from build123d import *

# Parameters (mm, degrees)
SKETCH_R     = 9
SKETCH_R_2   = 4
PAD_DEPTH    = 10
SKETCH001_R  = 2.5
POCKET_DEPTH = 10.001
CHAMFER_SIZE = 3


with BuildPart() as part:
    # Sketch → Pad (new body)
    with BuildSketch(Plane.XZ):
        with BuildLine():
            Line((0, 0), (0, 25))
            Line((0, 25), (-10, 25))
            Line((-10, 25), (-10, 55))
            Line((-10, 55), (0, 55))
            Line((0, 55), (0, 80))
            Line((0, 80), (-10, 80))
            Line((-10, 80), (-10, 110))
            Line((-10, 110), (0, 110))
            Line((0, 110), (0, 125))
            Line((0, 125), (-10.439, 125))
            ThreePointArc((-24.439, 139), (-20.338495, 129.100505), (-10.439, 125))
            Line((-24.439, 139), (-24.439, 151.456))
            ThreePointArc((12.872585, 161.471439), (-9.623992, 170.772207), (-24.439, 151.456))
            ThreePointArc((12.872585, 161.471439), (26.413305, 147.948816), (44.899018, 143))
            Line((44.899018, 143), (230, 143))
            Line((230, 143), (230, 131.156))
            Line((230, 131.156), (240, 131.156))
            Line((240, 131.156), (240, 101.156))
            Line((240, 101.156), (230, 101.156))
            Line((230, 101.156), (230, 61.156))
            Line((230, 61.156), (240, 61.156))
            Line((240, 61.156), (240, 31.156))
            Line((240, 31.156), (230, 31.156))
            Line((230, 31.156), (230, 25))
            ThreePointArc((230, 25), (219.393398, 20.606602), (215, 10))
            Line((215, 10), (211, 10))
            Line((211, 10), (211, 0))
            Line((211, 0), (131, 0))
            Line((131, 0), (131, 10))
            Line((131, 10), (80, 10))
            Line((80, 10), (80, 0))
            Line((80, 0), (0, 0))
        make_face()
        with Locations((15, 25)):
            Circle(SKETCH_R, mode=Mode.SUBTRACT)
        with Locations((-5.055, 150.4)):
            Circle(SKETCH_R_2, mode=Mode.SUBTRACT)
    extrude(amount=PAD_DEPTH)

    # Sketch001 → Pocket (cut, through all)
    with BuildSketch(Plane.XZ):
        with Locations((91.36, 135.87)):
            Circle(SKETCH001_R)
        with Locations((138.5, 135.87)):
            Circle(SKETCH001_R)
        with Locations((91.36, 88.73)):
            Circle(SKETCH001_R)
        with Locations((138.5, 88.73)):
            Circle(SKETCH001_R)
        with BuildLine():
            ThreePointArc((106.83, 129.542172), (114.93, 93.25), (123.03, 129.542172))
            Line((123.03, 129.542172), (123.03, 177.012172))
            Line((106.83, 177.012172), (123.03, 177.012172))
            Line((106.83, 129.542172), (106.83, 177.012172))
        make_face()
    extrude(amount=POCKET_DEPTH, mode=Mode.SUBTRACT)

    # Chamfer
    chamfer_edges = [part.edges().sort_by_distance(p)[0] for p in [
        (136, -10, 135.87),
        (88.86, -10, 88.73),
        (88.86, -10, 135.87),
        (136, -10, 88.73),
    ]]
    chamfer(chamfer_edges, length=CHAMFER_SIZE)


solid = part.part
Could you check a few things on this model? Use its own coordinates, in mm. A direction names the side the tool comes from. Round coordinates to 2 decimals unless told otherwise and drop trailing zeros. Write each loop counter-clockwise with the first axis right and the second up, starting at its lowest first coordinate (ties: lowest second). Pieces come first, ordered by that corner, then holes. Notation, with made-up numbers: (2, 31.25) -> (6, 31.25) arc R18 cw to (6, 41.25) -> close; hole circle Ø8 at (6.5, -40). An arc over 180 degrees is marked (long way). Use a Markdown table: item, result.
1. Please list where these lines run through material, in increasing order: probe 1 along Z at (x, y) = (91.36, -5); probe 2 along X at (y, z) = (-3.75, 88.73); probe 3 along Z at (x, y) = (138.5, -4.5).
Answer key:
| item | result |
|---|---|
| probe 1 | z = 10 to 86.23, 91.23 to 133.37, 138.37 to 143 |
| probe 2 | x = -10 to 88.86, 93.86 to 136, 141 to 230 |
| probe 3 | z = 0 to 86.23, 91.23 to 133.37, 138.37 to 143 |
2. Which directions (+Z, -Z, +X, -X, +Y, -Y) give clear straight access to the entire face, cutting with the end or side of a thin tool? Please do faces 1 (the face through (0, -5, 12)), 2 (the face through (-5, -5, 110)), 3 (the face through (75, -5, 143)).
Answer key:
| item | result |
|---|---|
| face 1 | -Z, -X, +Y, -Y |
| face 2 | -X, +Y, -Y |
| face 3 | +Z, +X, +Y, -Y |
3. If we section it at D-D (z = 157.5): List the corners of the cut face in (x, y) for me, then the cut area to 3 significant figures.
Answer key:
| item | result |
|---|---|
| outline | (-23.5, -10) -> (15.53, -10) -> (15.53, 0) -> (-23.5, 0) -> close |
| area | 390 mm^2 |
4. For pin 1 Ø3 at (y, z) = (-6, 5) entering from +X; pin 2 Ø2 at (x, y) = (53, -4.5) entering from -Z; pin 3 Ø5 at (x, y) = (174.5, -6.5) entering from +Z; pin 4 Ø4 at (y, z) = (-5.5, 128) entering from -X, each with a flat end and sliding along its axis, tell me the tip position at first contact or that it passes through.
Answer key:
| item | result |
|---|---|
| pin 1 | stops at x = 211 |
| pin 2 | stops at z = 0 |
| pin 3 | stops at z = 143 |
| pin 4 | stops at x = -21.16 |
5. We'd pull the mould along X, two halves only. Please class faces 4 (the face through (93.883, -7.146, 87.935)), 5 (the face through (235, -5, 131.156)), 6 (the face through (230, -5, 28)): +X half, -X half, draft (parallel to the pull), parting line (faces both ways), or undercut.
Answer key:
| item | result |
|---|---|
| face 4 | undercut |
| face 5 | draft |
| face 6 | +X half |
6. If we section it at B-B (x = 114.93): List the corners of the cut face in (y, z) for me.
Answer key:
| item | result |
|---|---|
| outline | (-10, 10) -> (0, 10) -> (0, 93.25) -> (-10, 93.25) -> close |
7. If we section it at C-C (y = -5.25): State how many separate pieces and enclosed holes the cut face has, then the cut area to 3 significant figures.
Answer key:
| item | result |
|---|---|
| separate pieces | 1 |
| enclosed holes | 6 |
| area | 33,000 mm^2 |
8. If we section it at A-A (z = 22): List the corners of the cut face in (x, y) for me.
Answer key:
| item | result |
|---|---|
| outline | (0, -10) -> (6.51, -10) -> (6.51, 0) -> (0, 0) -> close; (23.49, -10) -> (221, -10) -> (221, 0) -> (23.49, 0) -> close |
